from build123d import *

# Parameters (mm, degrees)
F0_W     = 24.5872
F0_H     = 38.1
F0_R     = 5.9436
F1_DEPTH = 6.35
F2_R     = 2.15265
F3_DEPTH = 24.5882


with BuildPart() as f1:
    # F0 (on Top) → F1 (new body)
    with BuildSketch(Plane.XY):
        with Locations((12.2936, 19.05)):
            Rectangle(F0_W, F0_H)
        with Locations((12.2936, 19.05)):
            Circle(F0_R, mode=Mode.SUBTRACT)
    extrude(amount=F1_DEPTH)

    # F2 (on face) → F3 (cut, through all)
    with BuildSketch(Plane(origin=(0, 0, 0), x_dir=(0, -1, 0), z_dir=(-1, 0, 0))):
        with Locations((-31.75, 3.175)):
            Circle(F2_R)
        with Locations((-6.35, 3.175)):
            Circle(F2_R)
    extrude(amount=-F3_DEPTH, mode=Mode.SUBTRACT)


solid = f1.part
Design review of the part built by this model. Coordinates are the model's own, in mm. Give positions to 0.01 mm unless a question says otherwise; leave off trailing zeros. Order: outer loops, then holes, each group sorted by start corner. A loop starts at its lowest first (then second) coordinate and runs counter-clockwise, first axis right, second up.
1. Mouldability with a two-part tool opening along Y and no side actions: class faces 1 (the flat face through (12, 38.1, 3)), 2 (the flat face through (18, 24, 0)), 3 (the cylindrical face through (12.1, 33.9, 3.3)) as +Y half, -Y half, draft (parallel to the pull), parting line (faces both ways), or undercut.
Solution:
face 1: +Y half
face 2: draft
face 3: undercut
2. To check wall thickness, follow L1, parallel to Y at x = 22.25, z = 3.25; L2, parallel to Y at x = 2, z = 4.25; L3, parallel to Z at x = 9.75, y = 31.75. State the ranges of each line that lie inside material, in increasing order.
Solution:
L1: y = 0 to 4.2, 8.5 to 29.6, 33.9 to 38.1
L2: y = 0 to 4.48, 8.22 to 29.88, 33.62 to 38.1
L3: z = 0 to 1.02, 5.33 to 6.35
3. Add section D-D, the plane x = 17.5. State the section outline as (y, z) points (3 decimals).
Solution:
outline: (0, 0) - (16.183, 0) - (16.183, 6.35) - (0, 6.35) - close; (21.917, 0) - (38.1, 0) - (38.1, 6.35) - (21.917, 6.35) - close; hole circle Ø4.305 at (6.35, 3.175); hole circle Ø4.305 at (31.75, 3.175)
4. Add section C-C, the plane y = 19.05. State the section outline as (x, z) points, then the cut area to 3 significant figures.
Solution:
outline: (0, 0) - (6.35, 0) - (6.35, 6.35) - (0, 6.35) - close; (18.24, 0) - (24.59, 0) - (24.59, 6.35) - (18.24, 6.35) - close
area: 80.6 mm2
5. For pin 1 Ø10.5 at (x, y) = (12.29, 19.05) entering from -Z, flat-tipped, find the tip position at first contact; note if it passes through.
Solution:
pin 1: passes through
6. Add section B-B, the plane z = 1.5. State the section outline as (x, y) points.
Solution:
outline: (0, 0) - (24.59, 0) - (24.59, 5) - (0, 5) - close; (0, 7.7) - (24.59, 7.7) - (24.59, 30.4) - (0, 30.4) - close; (0, 33.1) - (24.59, 33.1) - (24.59, 38.1) - (0, 38.1) - close; hole circle Ø11.89 at (12.29, 19.05)
7. Add section A-A, the plane x = 12.25. State the section outline as (y, z) points (3 decimals), then the cut area to 3 significant figures.
Solution:
outline: (0, 0) - (13.107, 0) - (13.107, 6.35) - (0, 6.35) - close; (24.993, 0) - (38.1, 0) - (38.1, 6.35) - (24.993, 6.35) - close; hole circle Ø4.305 at (6.35, 3.175); hole circle Ø4.305 at (31.75, 3.175)
area: 137 mm2
